Autodesk Inventor part; units mm, degrees
ref_plane "1_XY" through (0, 5.6896, 0) normal (0, 1, 0) x (1, 0, 0)
ref_plane "1_YZ" through (0, 5.6896, 0) normal (1, 0, 0) x (0, 0, -1)
ref_plane "1_ZX" through (0, 5.6896, 0) normal (0, 0, -1) x (0, 1, 0)
sketch "Sketch_1" plane through (0, 0, 0) normal (0, 0, 1) x (1, 0, 0)
  line L0 (-3.9497, 0) -> (-3.9497, -6.7945)
  line L1 (-3.9497, -6.7945) -> (-3.6957, -6.7945)
  line L2 (-3.6957, -6.7945) -> (-3.6957, -0.254)
  arc A0 (-3.4417, 0) -> (-3.6957, -0.254) centre (-3.4417, -0.254) ccw
  line L3 (-3.4417, 0) -> (3.4417, 0)
  arc A1 (3.6957, -0.254) -> (3.4417, 0) centre (3.4417, -0.254) ccw
  line L4 (3.6957, -0.254) -> (3.6957, -6.7945)
  line L5 (3.6957, -6.7945) -> (3.9497, -6.7945)
  line L6 (3.9497, -6.7945) -> (3.9497, 0)
  arc A2 (3.9497, 0) -> (3.6957, 0.254) centre (3.6957, 0) ccw
  line L7 (3.6957, 0.254) -> (-3.6957, 0.254)
  arc A3 (-3.6957, 0.254) -> (-3.9497, 0) centre (-3.6957, 0) ccw
extrude "Extrusion1" add sketch "Sketch_1" along normal mid plane 13.0048
sketch "Sketch_2" plane through (0, 0, 0) normal (1, 0, 0) x (0, 1, 0)
  line L0 (0, 7.8029) -> (-9.398, 7.8029)
  line L1 (-9.398, 7.8029) -> (-9.398, -7.8029)
  line L2 (-9.398, -7.8029) -> (0, -7.8029)
  line L3 (0, -7.8029) -> (0, -5.0927)
  line L4 (0, -5.0927) -> (-6.3246, -5.0927)
  line L5 (-6.3246, -5.0927) -> (-6.3246, -2.7305)
  line L6 (-6.3246, -2.7305) -> (-6.6675, -2.7305)
  arc A0 (-6.7945, -2.6035) -> (-6.6675, -2.7305) centre (-6.6675, -2.6035) ccw
  line L7 (-6.7945, -2.6035) -> (-6.7945, -2.0955)
  arc A1 (-6.6675, -1.9685) -> (-6.7945, -2.0955) centre (-6.6675, -2.0955) ccw
  line L8 (-6.6675, -1.9685) -> (-6.3246, -1.9685)
  line L9 (-6.3246, -1.9685) -> (-6.3246, 1.9685)
  line L10 (-6.3246, 1.9685) -> (-6.6675, 1.9685)
  arc A2 (-6.7945, 2.0955) -> (-6.6675, 1.9685) centre (-6.6675, 2.0955) ccw
  line L11 (-6.7945, 2.0955) -> (-6.7945, 2.6035)
  arc A3 (-6.6675, 2.7305) -> (-6.7945, 2.6035) centre (-6.6675, 2.6035) ccw
  line L12 (-6.6675, 2.7305) -> (-6.3246, 2.7305)
  line L13 (-6.3246, 2.7305) -> (-6.3246, 5.0927)
  line L14 (-6.3246, 5.0927) -> (0, 5.0927)
  line L15 (0, 5.0927) -> (0, 7.8029)
extrude "Extrusion2" cut sketch "Sketch_2" along normal mid plane 7.8994
sketch "Sketch_7" plane through (0, 0, 0) normal (0, 0, 1) x (1, 0, 0)
  line L0 (0, 0.127) -> (0, 7.493)
  line L1 (0, 7.493) -> (2.479, 7.493)
  line L2 (2.479, 7.493) -> (3.0988, 6.8732)
  line L3 (3.0988, 6.8732) -> (3.0988, 1.397)
  line L4 (3.0988, 1.397) -> (4.0005, 1.397)
  line L5 (4.0005, 1.397) -> (4.0005, 0.508)
  line L6 (4.0005, 0.508) -> (3.2537, 0.508)
  line L7 (3.2537, 0.508) -> (3.2537, 0.127)
  line L8 (3.2537, 0.127) -> (0, 0.127)
  line L9 (0, 0.127) -> (0, 7.493)
revolve "Revolution1" add sketch "Sketch_7" angle 360 about axis through (0, 0.127, 0) along (0, -1, 0)
sketch "Sketch_8" plane through (0, 0.254, 0) normal (0, 1, 0) x (1, 0, 0)
  line L0 (-0.3937, 2.4892) -> (0.3937, 2.4892)
  line L1 (0.3937, 2.4892) -> (0.3937, 10.4902)
  line L2 (0.3937, 10.4902) -> (-0.3937, 10.4902)
  line L3 (-0.3937, 10.4902) -> (-0.3937, 2.4892)
extrude "Extrusion3" cut sketch "Sketch_8" along normal blind 7.8232
sketch "Sketch5" plane through (-3.9497, 0, -6.5024) normal (0, -1, 0) x (1, 0, 0)
  point P0 (3.9497, 6.5024)
hole "Drilling 1" at (0, 0, 0) direction (0, 1, 0) diameter 4.3383 depth 7.747
ref_plane "1_XY" through (0, 5.6896, 0) normal (0, 1, 0) x (1, 0, 0)
ref_plane "1_YZ" through (0, 5.6896, 0) normal (1, 0, 0) x (0, 0, -1)
ref_plane "1_ZX" through (0, 5.6896, 0) normal (0, 0, -1) x (0, 1, 0)
ref_plane "2_XY" through (0, 4.2672, 0) normal (0, 1, 0) x (1, 0, 0)
ref_plane "2_YZ" through (0, 4.2672, 0) normal (1, 0, 0) x (0, 0, -1)
ref_plane "2_ZX" through (0, 4.2672, 0) normal (0, 0, -1) x (0, 1, 0)
ref_plane "3_XY" through (0, 2.8448, 0) normal (0, 1, 0) x (1, 0, 0)
ref_plane "3_YZ" through (0, 2.8448, 0) normal (1, 0, 0) x (0, 0, -1)
ref_plane "3_ZX" through (0, 2.8448, 0) normal (0, 0, -1) x (0, 1, 0)
ref_plane "4_XY" through (0, 1.778, 0) normal (0, 1, 0) x (1, 0, 0)
ref_plane "4_YZ" through (0, 1.778, 0) normal (1, 0, 0) x (0, 0, -1)
ref_plane "4_ZX" through (0, 1.778, 0) normal (0, 0, -1) x (0, 1, 0)
ref_plane "to_base_XY" through (0, 0, 0) normal (0, 1, 0) x (1, 0, 0)
ref_plane "to_base_YZ" through (0, 0, 0) normal (1, 0, 0) x (0, 0, -1)
ref_plane "to_base_ZX" through (0, 0, 0) normal (0, 0, -1) x (0, 1, 0)
properties part number "M201A2M201BR-bushing"
Here's how the part is built. I have some questions about the finished solid (model axes, mm). A direction names the side the tool comes from. Give positions to 0.01 mm unless a question says otherwise; leave off trailing zeros. Write each loop counter-clockwise with the first axis right and the second up, starting at its lowest first coordinate (ties: lowest second). Pieces come first, ordered by that corner, then holes. Notation, with made-up numbers: (42.5, 62) -> (87.5, 62) arc R26 cw to (87.5, 78) -> close; hole circle Ø9 at (-34, 4.5). An arc over 180 degrees is marked (long way). Write each question's results on one line, items separated by ' | '.
Item 1: On a 3-axis mill with a long thin cutter (end or side, diameter ignored), from which of +Z, -Z, +X, -X, +Y, -Y can I reach the whole of each face in a straight line? I mean faces 1 (the face through (-2, 0.508, -3)), 2 (the face through (-0.65, 3.8, -2.07)), 3 (the face through (-3.696, -4, 0)), 4 (the face through (0, 1, 4)), 5 (the face through (-0.394, 3, -2.9)). Say none if no direction works.
Output:
face 1: none | face 2: +Y, -Y | face 3: +Z, -Z, -Y | face 4: +Y | face 5: -Z, +Y
Item 2: If I drill on L1, parallel to X at y = -0.75, z = -1; L2, parallel to X at y = 3, z = 0; L3, parallel to Y at x = 0, z = -5, over which ranges is the centre line in solid material (lowest first)?
Output:
L1: x = -3.95 to -3.7, 3.7 to 3.95 | L2: x = -3.1 to -2.17, 2.17 to 3.1 | L3: y = 0 to 0.25
Item 3: We'd pull the mould along X, two halves only. Please class faces 6 (the face through (2, 1.397, 3)), 7 (the face through (-3.95, -3, 0)), 8 (the face through (3.696, -3, 0)): pulls with the +X half, pulls with the -X half, needs draft (parallel to the pull), parting line crosses it, or undercut.
Output:
face 6: needs draft | face 7: pulls with the -X half | face 8: undercut
Item 4: For pin 1 Ø1 at (x, y) = (0.5, 4.5) entering from +Z; pin 2 Ø0.9 at (x, y) = (0, 2) entering from -Z; pin 3 Ø2 at (x, z) = (2, 0) entering from -Y, each with a flat end and sliding along its axis, tell me the tip position at first contact or that it passes through.
Output:
pin 1: stops at z = 3.1 | pin 2: stops at z = -3.07 | pin 3: stops at y = 0
Item 5: Suppose I cut it at D-D on y = 1.75. Write out the boundary of the cut face in (x, z), plus the area to 3 significant figures.
Output:
outline: (-0.39, -3.07) -> (-0.39, -2.49) -> (0.39, -2.49) -> (0.39, -3.07) arc R3.1 ccw (long way) to start; hole circle Ø4.34 at (0, 0) | area: 14.9 mm^2
Item 6: Suppose I cut it at A-A on y = -2.25. Write out the boundary of the cut face in (x, z).
Output:
outline: (-3.95, -5.09) -> (-3.7, -5.09) -> (-3.7, 5.09) -> (-3.95, 5.09) -> close; (3.7, -5.09) -> (3.95, -5.09) -> (3.95, 5.09) -> (3.7, 5.09) -> close
